Source: three-view drawing plus pictorial views. Frame: mm from the lowest corner of the part. A direction names the side the tool comes from. Give positions to 0.01 mm unless a question says otherwise; leave off trailing zeros. Order: outer loops, then holes, each group sorted by start corner. A loop starts at its lowest first (then second) coordinate and runs counter-clockwise, first axis right, second up. Notation, with made-up numbers: (-10.5, 74.5) - (-1.5, 74.5) arc R22 ccw to (-1.5, 107.5) - close; hole circle Ø3 at (-9.75, 2). An arc over 180 degrees is marked (long way). Answer in a Markdown table with one row per item. Add a question column.
1. Section query A-A on z = 2.5. Return loops of the section in (x, y), and give its area (3 significant figures).
2. Mould query, pull axis X, two halves, no side actions, for the marked faces 4, 5, 6 and 7. Classes: released by +X, released by -X, zero draft, split by the parting line, or undercut.
3. Access query for the marked faces 1, 2 and 3. Directions: +Z, -Z, +X, -X, +Y, -Y. A direction counts if a zero-diameter tool reaches every point of the face in a straight line with its end or side. Return the directions, or none.
4. Contact query for flat-ended pins moving along their axis: pin 1 (3 mm diameter, centred on y = 2.5, z = 3.5, fed in from +X); pin 2 (1.9 mm diameter, centred on y = 4, z = 3.5, fed in from -X); pin 3 (1.9 mm diameter, centred on x = 21.5, z = 4.5, fed in from -Y). Output: stop coordinate, or through.
5. Ray query, line 1 (X direction, y = 51, z = 4.5); line 2 (X direction, y = 3.5, z = 6); line 3 (Y direction, x = 11.5, z = 5.5). Return the intervals inside material, ascending. Write a range as [from, to].
6. Section query B-B on x = 51.5. Return loops of the section in (y, z).
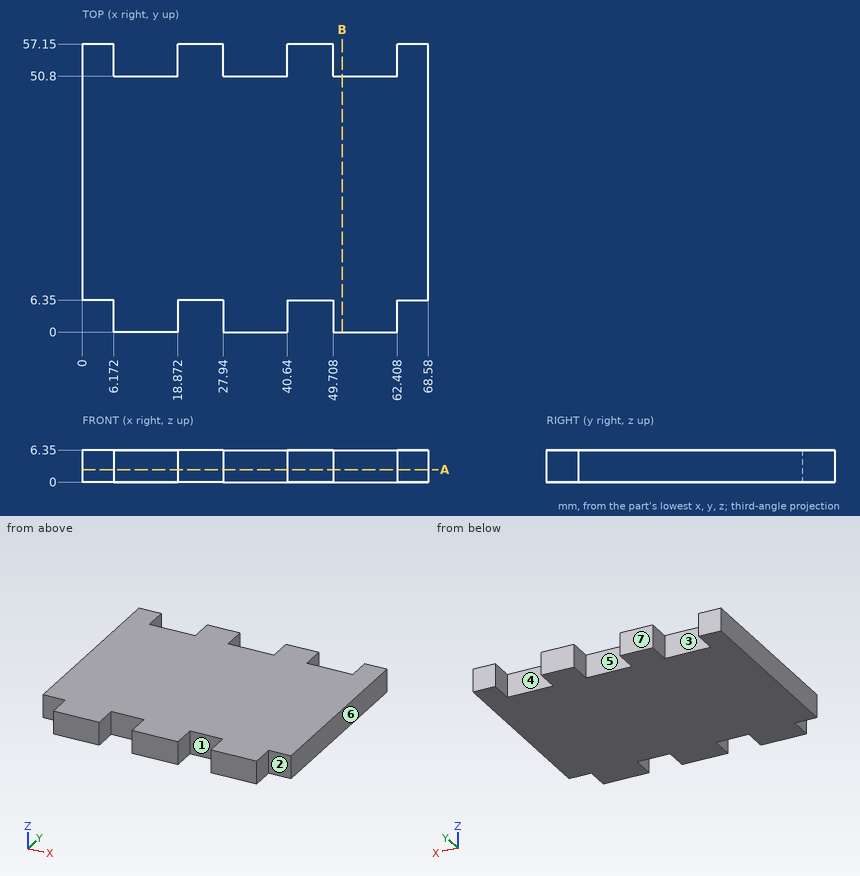
Answer:
| question | item | result |
|---|---|---|
| 1 | outline | (0, 6.35) - (6.17, 6.35) - (6.17, 0) - (18.87, 0) - (18.87, 6.35) - (27.94, 6.35) - (27.94, 0) - (40.64, 0) - (40.64, 6.35) - (49.71, 6.35) - (49.71, 0) - (62.41, 0) - (62.41, 6.35) - (68.58, 6.35) - (68.58, 57.15) - (62.41, 57.15) - (62.41, 50.8) - (49.71, 50.8) - (49.71, 57.15) - (40.64, 57.15) - (40.64, 50.8) - (27.94, 50.8) - (27.94, 57.15) - (18.87, 57.15) - (18.87, 50.8) - (6.17, 50.8) - (6.17, 57.15) - (0, 57.15) - close |
| 1 | area | 3,480 mm² |
| 2 | face 4 | undercut |
| 2 | face 5 | undercut |
| 2 | face 6 | released by +X |
| 2 | face 7 | zero draft |
| 3 | face 1 | +Z, -Z, -Y |
| 3 | face 2 | +Z, -Z, +X, -Y |
| 3 | face 3 | +Z, -Z, +Y |
| 4 | pin 1 | stops at x = 62.41 |
| 4 | pin 2 | stops at x = 6.17 |
| 4 | pin 3 | stops at y = 6.35 |
| 5 | line 1 | x = [0, 6.17], [18.87, 27.94], [40.64, 49.71], [62.41, 68.58] |
| 5 | line 2 | x = [6.17, 18.87], [27.94, 40.64], [49.71, 62.41] |
| 5 | line 3 | y = [0, 50.8] |
| 6 | outline | (0, 0) - (50.8, 0) - (50.8, 6.35) - (0, 6.35) - close |
